Could you check a few things on this model? Use its own coordinates, in mm. Round coordinates to 2 decimals unless told otherwise and drop trailing zeros. Loops run counter-clockwise (first coordinate to the right, second up) from the corner with the lowest first, then second, coordinate; pieces in that order, holes last. Notation, with made-up numbers: (11.5, 38) -> (69.5, 38) arc R28 ccw to (69.5, 68) -> close; hole circle Ø3 at (30, 79). An arc over 180 degrees is marked (long way). One line per item, written item: value.
from build123d import *

# Parameters (mm, degrees)
F0_W     = 30
F0_H     = 75
F1_DEPTH = 2
F2_R     = 5.08
F3_W     = 26.70412
F3_H     = 34.643184
F4_DEPTH = 0.1524


with BuildPart() as f1:
    # F0 (on Front) → F1 (new body)
    with BuildSketch(Plane.XZ):
        with Locations((15, 37.5)):
            Rectangle(F0_W, F0_H)
    extrude(amount=F1_DEPTH)

    # F2
    f2_edges = [f1.edges().sort_by_distance(p)[0] for p in [
        (30, -1, 75),
        (0, -1, 75),
    ]]
    fillet(f2_edges, radius=F2_R)

    # F3 (on face) → F4 (cut)
    with BuildSketch(Plane.XZ.offset(2)):
        with Locations((15.126201, 19.738285)):
            Rectangle(F3_W, F3_H)
    extrude(amount=-F4_DEPTH, mode=Mode.SUBTRACT)


solid = f1.part
(1) If I drill on L1, parallel to Z at x = 16.75, y = -1.9; L2, parallel to Y at x = 16.5, z = 3.5; L3, parallel to Z at x = 28, y = -1.65, over which ranges is the centre line in solid material (lowest first)?
Recorded:
L1: 0 to 2.42, 37.06 to 75
L2: -1.85 to 0
L3: 0 to 73.96
(2) If we section it at A-A, the plane z = 23: Please give me the cut outline in (x, y), then the cut area to 3 significant figures.
Recorded:
outline: (0, -2) -> (1.77, -2) -> (1.77, -1.85) -> (28.48, -1.85) -> (28.48, -2) -> (30, -2) -> (30, 0) -> (0, 0) -> close
area: 55.9 mm²
(3) Thinking about a two-plate mould opening in X: for faces 1 (the face through (0, -1, 34)), 2 (the face through (15, -1.848, 20)), 3 (the face through (30, -1, 34)), 4 (the face through (15, 0, 38)), which applies, released by +X, released by -X, zero draft, split by the parting line, or undercut?
Recorded:
face 1: released by -X
face 2: undercut
face 3: released by +X
face 4: zero draft
(4) If we section it at B-B, the plane x = 21: Please give me the cut outline in (y, z), then the cut area to 3 significant figures.
Recorded:
outline: (-2, 0) -> (0, 0) -> (0, 75) -> (-2, 75) -> (-2, 37.06) -> (-1.85, 37.06) -> (-1.85, 2.42) -> (-2, 2.42) -> close
area: 145 mm²
(5) I'm going to push a flat-ended pin straight in: pin 1 Ø8 at (x, z) = (12.5, 11.5) entering from -Y. Where does the tip first touch, or does it pass through?
Recorded:
pin 1: y = -1.85
